Part model, mm, in its own coordinate system. Round coordinates to 2 decimals unless told otherwise and drop trailing zeros. Loops run counter-clockwise (first coordinate to the right, second up) from the corner with the lowest first, then second, coordinate; pieces in that order, holes last.
Autodesk Inventor part; units mm, degrees
ref_plane "YZ Plane" through (0, 0, 0) normal (1, 0, 0) x (0, 1, 0)
ref_plane "XZ Plane" through (0, 0, 0) normal (0, 1, 0) x (-1, 0, 0)
ref_plane "XY Plane" through (0, 0, 0) normal (0, 0, 1) x (1, 0, 0)
sketch "Sketch1" plane through (0, 0, 0) normal (1, 0, 0) x (0, 1, 0)
  line L0 (-0.4142, 8.5) -> (-1, 9.0858)
  line L1 (-1, 9.0858) -> (-1, 9.9142)
  line L2 (-1, 9.9142) -> (-0.4142, 10.5)
  line L3 (-0.4142, 10.5) -> (0.4142, 10.5)
  line L4 (0.4142, 10.5) -> (1, 9.9142)
  line L5 (1, 9.9142) -> (1, 9.0858)
  line L6 (1, 9.0858) -> (0.4142, 8.5)
  line L7 (0.4142, 8.5) -> (-0.4142, 8.5)
  line L8 (3.1428, 0) -> (-2.1354, 0)
  point P0 (0, 0)
  point P1 (0, 9.5)
  dimension "d2" = 2
  dimension "d3" = 0
  dimension "d5" = 8.5
revolve "Revolution1" add sketch "Sketch1" angle 360 about axis through (0, 3.1428, 0) along (0, -1, 0)
properties part number "Ring"
1) Wall check: line 1 along Z through (x, y) = (0, 0); line 2 along X through (y, z) = (0.5, 3). Give the ranges that are in metal, low to high.
Values:
line 1: z = -10.5 to -8.5, 8.5 to 10.5
line 2: x = -9.97 to -8.04, 8.04 to 9.97
2) Mould opens along X. For faces 1 (the face through (3.2, 0, 10)), 2 (the face through (3, 1, 9)), 3 (the face through (-7.167, -0.006, 4.57)) say: released by +X, released by -X, zero draft, split by the parting line, or undercut.
Values:
face 1: split by the parting line
face 2: zero draft
face 3: undercut
3) Slice it at B-B, the plane x = 0. Give the cut face in (y, z).
Values:
outline: (-1, -9.91) - (-0.41, -10.5) - (0.41, -10.5) - (1, -9.91) - (1, -9.09) - (0.41, -8.5) - (-0.41, -8.5) - (-1, -9.09) - close; (-1, 9.09) - (-0.41, 8.5) - (0.41, 8.5) - (1, 9.09) - (1, 9.91) - (0.41, 10.5) - (-0.41, 10.5) - (-1, 9.91) - close
4) Slice it at A-A, the plane z = 0. Give the cut face in (x, y).
Values:
outline: (-10.5, -0.41) - (-9.91, -1) - (-9.09, -1) - (-8.5, -0.41) - (-8.5, 0.41) - (-9.09, 1) - (-9.91, 1) - (-10.5, 0.41) - close; (8.5, -0.41) - (9.09, -1) - (9.91, -1) - (10.5, -0.41) - (10.5, 0.41) - (9.91, 1) - (9.09, 1) - (8.5, 0.41) - close
5) Slice it at C-C, the plane y = 0.05. Give the cut face in (x, z), then the cut area to 3 significant figures.
Values:
outline: circle Ø21 at (0, 0); hole circle Ø17 at (0, 0)
area: 119 mm2
